Source: three-view drawing plus pictorial views. Frame: mm from the lowest corner of the part. Round coordinates to 2 decimals unless told otherwise and drop trailing zeros. Write each loop counter-clockwise with the first axis right and the second up, starting at its lowest first coordinate (ties: lowest second). Pieces come first, ordered by that corner, then holes. Notation, with made-up numbers: M -24.5,-9 L -7.5,-9 A18 cw -7.5,8 Z; hole C 21.5,-35.75 d6. An arc over 180 degrees is marked long. Answer in a Markdown table with one row per item.
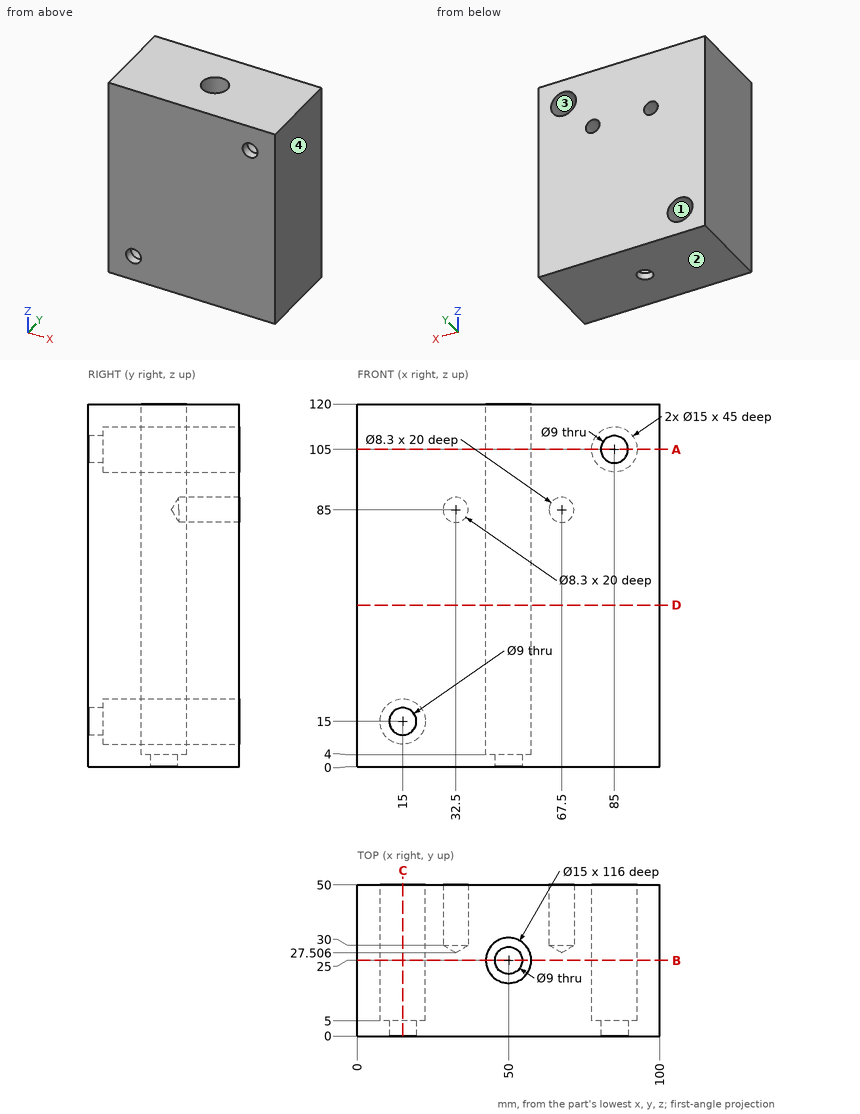
Q1. Pull-direction query (X, two-part tool) for the marked faces 1, 2, 3 and 4; classes: pulls with the +X half, pulls with the -X half, needs draft (parallel to the pull), parting line crosses it, or undercut.
Solutions:
| item | result |
|---|---|
| face 1 | undercut |
| face 2 | needs draft |
| face 3 | undercut |
| face 4 | pulls with the +X half |
Q2. Section D-D (z = 53.5). Return loops of the section in (x, y), and give its area (3 significant figures).
Solutions:
| item | result |
|---|---|
| outline | M 0,0 L 100,0 L 100,50 L 0,50 Z; hole C 50,25 d15 |
| area | 4,820 mm2 |
Q3. Material intervals for probe 1 along X at (y, z) = (45, 85); probe 2 along X at (y, z) = (1, 105); probe 3 along Z at (x, y) = (15, 1), sorted ascending.
Solutions:
| item | result |
|---|---|
| probe 1 | x = 0 to 28.35, 36.65 to 63.35, 71.65 to 100 |
| probe 2 | x = 0 to 80.5, 89.5 to 100 |
| probe 3 | z = 0 to 10.5, 19.5 to 120 |
Q4. Section C-C (x = 15). Return loops of the section in (y, z), and give its area (3 significant figures).
Solutions:
| item | result |
|---|---|
| outline | M 0,0 L 50,0 L 50,7.5 L 5,7.5 L 5,10.5 L 0,10.5 Z; M 0,19.5 L 5,19.5 L 5,22.5 L 50,22.5 L 50,120 L 0,120 Z |
| area | 5,280 mm2 |
Q5. Section B-B (y = 25). Return loops of the section in (x, z).
Solutions:
| item | result |
|---|---|
| outline | M 0,0 L 45.5,0 L 45.5,4 L 42.5,4 L 42.5,120 L 0,120 Z; M 54.5,0 L 100,0 L 100,120 L 57.5,120 L 57.5,4 L 54.5,4 Z; hole C 15,15 d15; hole C 85,105 d15 |
Q6. Contact query for flat-ended pins moving along their axis: pin 1 Ø1.5 at (y, z) = (20.5, 89.5) entering from -X; pin 2 Ø7.5 at (x, z) = (67.5, 85) entering from +Y; pin 3 Ø4.5 at (x, y) = (53.5, 28.5) entering from +Z; pin 4 Ø10.5 at (x, z) = (15, 15) entering from +Y. Output: stop coordinate, or through.
Solutions:
| item | result |
|---|---|
| pin 1 | stops at x = 0 |
| pin 2 | stops at y = 29.76 |
| pin 3 | stops at z = 4 |
| pin 4 | stops at y = 5 |
Q7. Section A-A (z = 105). Return loops of the section in (x, y).
Solutions:
| item | result |
|---|---|
| outline | M 0,0 L 80.5,0 L 80.5,5 L 77.5,5 L 77.5,50 L 0,50 Z; M 89.5,0 L 100,0 L 100,50 L 92.5,50 L 92.5,5 L 89.5,5 Z; hole C 50,25 d15 |
